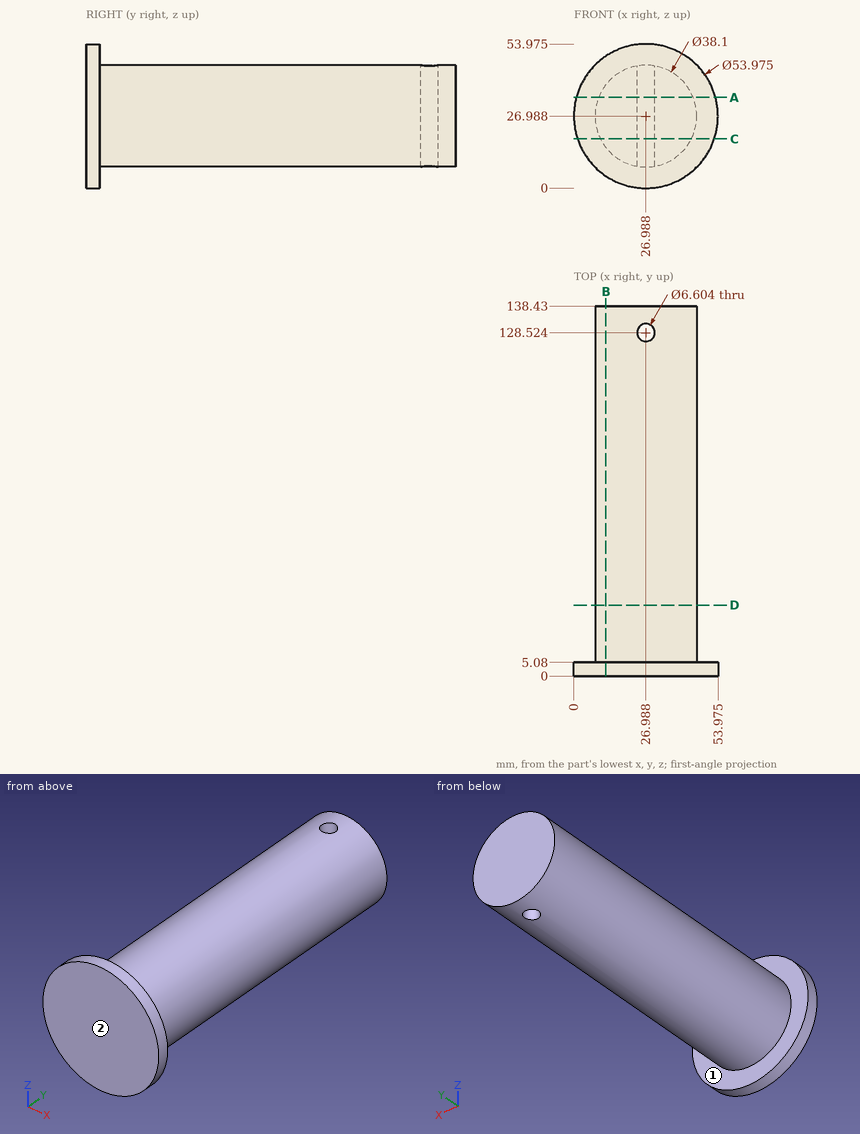
The figure shows three views and two pictorial views of one solid part (mm, origin at its lowest corner). Answer the questions. A direction names the side the tool comes from. Round coordinates to 2 decimals unless told otherwise and drop trailing zeros. Loops run counter-clockwise (first coordinate to the right, second up) from the corner with the lowest first, then second, coordinate; pieces in that order, holes last. Notation, with made-up numbers: (-22, -12) -> (5, -12) arc R16 ccw to (5, 13) -> close; hole circle Ø7 at (4.5, 85). An arc over 180 degrees is marked (long way). Use one line per item in the form item = value.
(1) Straight lines are drawn through the part: line 1 (X direction, y = 125, z = 27.5) (1 decimal); line 2 (Y direction, x = 7, z = 24); line 3 (X direction, y = 129.5, z = 36) (1 decimal). For each, find the intervals that lie inside material, in ascending order.
Answer list:
line_1 = 7.9 to 46
line_2 = 0 to 5.08
line_3 = 10.2 to 23.8, 30.1 to 43.8
(2) Find section C-C on z = 18.5. Give the vertices of the cut face in (x, y) (1 decimal).
Answer list:
outline = (1.4, 0) -> (52.6, 0) -> (52.6, 5.1) -> (44, 5.1) -> (44, 138.4) -> (9.9, 138.4) -> (9.9, 5.1) -> (1.4, 5.1) -> close; hole circle Ø6.6 at (27, 128.5)
(3) Find section A-A on z = 34. Give the vertices of the cut face in (x, y) (1 decimal), then the cut area to 3 significant figures.
Answer list:
outline = (0.9, 0) -> (53, 0) -> (53, 5.1) -> (44.7, 5.1) -> (44.7, 138.4) -> (9.3, 138.4) -> (9.3, 5.1) -> (0.9, 5.1) -> close; hole circle Ø6.6 at (27, 128.5)
area = 4,950 mm2
(4) A tool of negligible diameter and unlimited length cuts with its end or side. For the marked faces 1 and 2, from which of +Z, -Z, +X, -X, +Y, -Y can it reach the whole face along a straight path? Write none if from no direction.
Answer list:
face_1 = +Y
face_2 = +Z, -Z, +X, -X, -Y
(5) Flat-ended cylindrical pins translate along their axes: P1, Ø6, axis at x = 17.5, y = 123.5, coming from the +Z side; P2, Ø1, axis at y = 62, z = 37, coming from the -X side; P3, Ø1.5, axis at x = 34, y = 21, coming from the -Z side; P4, Ø5.5, axis at x = 26.99, y = 128.52, coming from the -Z side. Find the tip coordinate at first contact, or state that the pin passes through.
Answer list:
P1 = 44.9
P2 = 10.48
P3 = 9
P4 = through
(6) Find section D-D on y = 26.5. Give the vertices of the cut face in (x, z).
Answer list:
outline = circle Ø38.1 at (26.99, 26.99)
(7) Find section B-B on x = 12. Give the vertices of the cut face in (y, z) (1 decimal), then the cut area to 3 significant figures.
Answer list:
outline = (0, 4.5) -> (5.1, 4.5) -> (5.1, 15.2) -> (138.4, 15.2) -> (138.4, 38.7) -> (5.1, 38.7) -> (5.1, 49.4) -> (0, 49.4) -> close
area = 3,360 mm2
